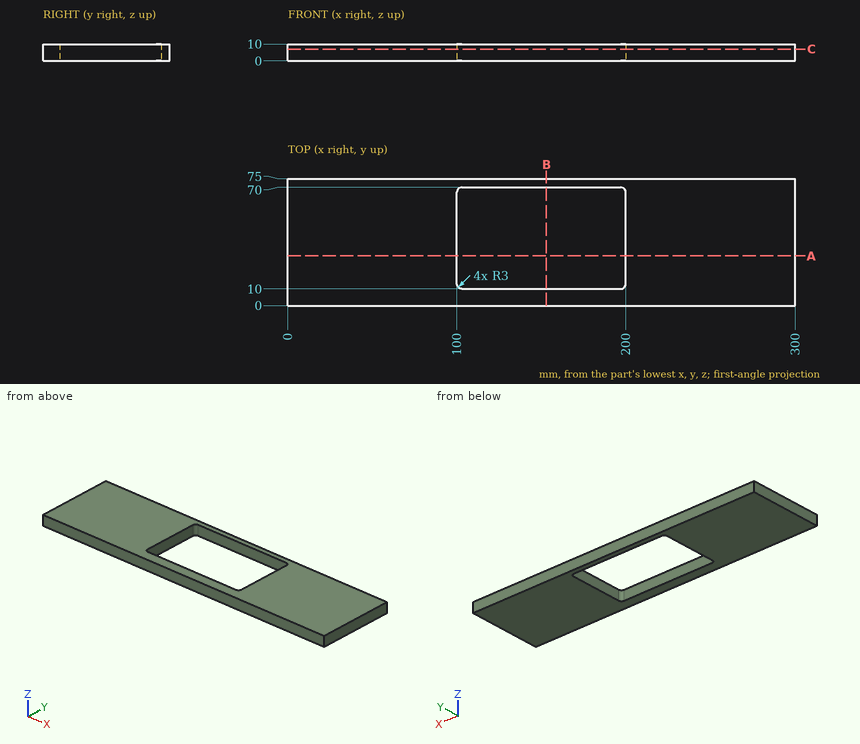
Geometry: see drawing. Coordinates: mm, zero at the bounding-box minimum. Give positions to 0.01 mm unless a question says otherwise; leave off trailing zeros. Order: outer loops, then holes, each group sorted by start corner. A loop starts at its lowest first (then second) coordinate and runs counter-clockwise, first axis right, second up. Notation, with made-up numbers: (60.5, -14) - (69.5, -14) arc R22 cw to (69.5, 19) - close; hole circle Ø9 at (72, 76.5). An arc over 180 degrees is marked (long way). Use a Markdown table: item, result.
(1) Section query C-C (z = 7). Output: boundary loops of the cut face in (x, y).
Computed values:
| item | result |
|---|---|
| outline | (0, 0) - (300, 0) - (300, 75) - (0, 75) - close; hole (100, 13) arc R3 ccw to (103, 10) - (197, 10) arc R3 ccw to (200, 13) - (200, 67) arc R3 ccw to (197, 70) - (103, 70) arc R3 ccw to (100, 67) - close |
(2) Line query: line 1 (Y direction, x = 105.5, z = 9.25); line 2 (X direction, y = 63, z = 2); line 3 (Y direction, x = 100.5, z = 8.75). Output: solid intervals per line, ascending. Write a range as from..to.
Computed values:
| item | result |
|---|---|
| line 1 | y = 0..10, 70..75 |
| line 2 | x = 0..100, 200..300 |
| line 3 | y = 0..11.34, 68.66..75 |
(3) Section query A-A (y = 29.5). Output: boundary loops of the cut face in (x, z).
Computed values:
| item | result |
|---|---|
| outline | (0, 0) - (100, 0) - (100, 10) - (0, 10) - close; (200, 0) - (300, 0) - (300, 10) - (200, 10) - close |
(4) Section query B-B (x = 153). Output: boundary loops of the cut face in (y, z), then the cut area to 3 significant figures.
Computed values:
| item | result |
|---|---|
| outline | (0, 0) - (10, 0) - (10, 10) - (0, 10) - close; (70, 0) - (75, 0) - (75, 10) - (70, 10) - close |
| area | 150 mm2 |
